The drawing under review shows one solid part. Ordinate dimensions are in mm from its lowest x, y, z. A direction names the side the tool comes from. Give positions to 0.01 mm unless a question says otherwise; leave off trailing zeros. Loops run counter-clockwise (first coordinate to the right, second up) from the corner with the lowest first, then second, coordinate; pieces in that order, holes last.
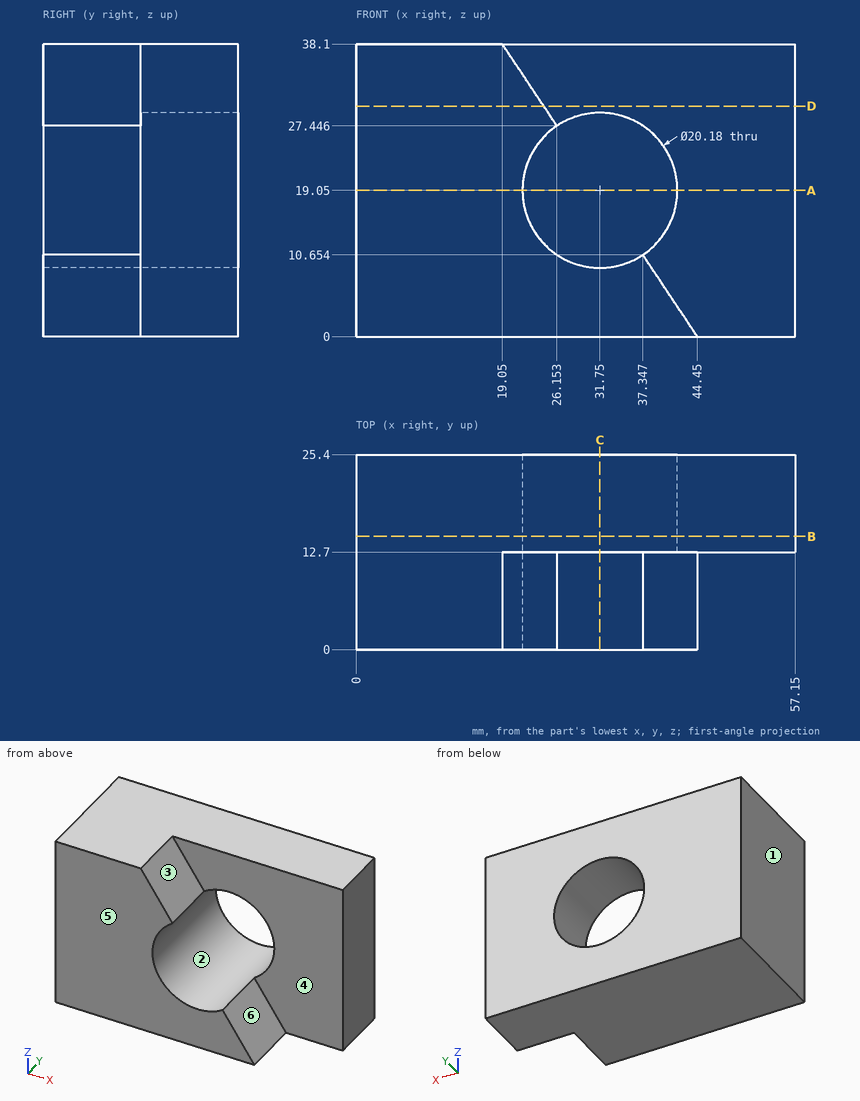
Item 1: Tool access review of the marked faces 5 and 6: name each direction out of +Z, -Z, +X, -X, +Y, -Y from which nothing blocks a thin tool from reaching the whole face with its end or side.
Answer:
face 5: +Z, -Z, +X, -X, -Y
face 6: +Z, +X, -Y
Item 2: Take a section at B-B on y = 14.75. Give the boundary of the cut face in (x, z).
Answer:
outline: (0, 0) - (57.15, 0) - (57.15, 38.1) - (0, 38.1) - close; hole circle Ø20.18 at (31.75, 19.05)
Item 3: Clearance check with flat-ended pins moving along their axes: pin 1 Ø8 at (y, z) = (12, 4) entering from -X; pin 2 Ø11.5 at (x, z) = (36.5, 27.5) entering from -Y; pin 3 Ø12 at (x, z) = (31.75, 19.05) entering from +Y. State where each tip first meets the part, or that it passes through.
Answer:
pin 1: stops at x = 0
pin 2: stops at y = 12.7
pin 3: passes through
Item 4: Take a section at D-D on z = 30. Give the boundary of the cut face in (x, y).
Answer:
outline: (0, 0) - (24.45, 0) - (24.45, 12.7) - (57.15, 12.7) - (57.15, 25.4) - (0, 25.4) - close
Item 5: For L1, parallel to X at y = 15.75, z = 19.05; L2, parallel to Z at x = 31.75, y = 15.5; L3, parallel to Y at x = 30.5, z = 35, list the stretches that pass through material, from the lowest coordinate up.
Answer:
L1: x = 0 to 21.66, 41.84 to 57.15
L2: z = 0 to 8.96, 29.14 to 38.1
L3: y = 12.7 to 25.4
Item 6: The part is to be moulded in two halves that separate along X. For the marked faces 1, 2, 3 and 4, say which applies: released by +X, released by -X, zero draft, split by the parting line, or undercut.
Answer:
face 1: released by -X
face 2: undercut
face 3: released by +X
face 4: zero draft
Item 7: Take a section at C-C on x = 31.75. Give the boundary of the cut face in (y, z), and give its area (3 significant figures).
Answer:
outline: (0, 0) - (25.4, 0) - (25.4, 8.96) - (0, 8.96) - close; (12.7, 29.14) - (25.4, 29.14) - (25.4, 38.1) - (12.7, 38.1) - close
area: 341 mm2
Item 8: Take a section at A-A on z = 19.05. Give the boundary of the cut face in (x, y).
Answer:
outline: (0, 0) - (21.66, 0) - (21.66, 25.4) - (0, 25.4) - close; (41.84, 12.7) - (57.15, 12.7) - (57.15, 25.4) - (41.84, 25.4) - close
